For this review, take the finished solid that the model builds, in its own axes (mm). A direction names the side the tool comes from. Round coordinates to 2 decimals unless told otherwise and drop trailing zeros. Order: outer loops, then holes, each group sorted by start corner. A loop starts at its lowest first (then second) coordinate and runs counter-clockwise, first axis right, second up. Notation, with made-up numbers: M 82.5,34 L 121.5,34 A23 cw 121.5,62 Z; hole C 14,21 d4. An arc over 180 degrees is marked long. Put each result on its own line as item: value.
Autodesk Inventor part; units mm, degrees
ref_plane "YZ Plane" through (0, 0, 0) normal (1, 0, 0) x (0, 1, 0)
ref_plane "XZ Plane" through (0, 0, 0) normal (0, 1, 0) x (-1, 0, 0)
ref_plane "XY Plane" through (0, 0, 0) normal (0, 0, 1) x (1, 0, 0)
sketch "Sketch1" plane through (0, 0, 0) normal (1, 0, 0) x (0, 1, 0)
  line L0 (27.1, -22.6) -> (-27.1, -22.6)
  line L1 (-27.1, -22.6) -> (-27.1, 22.6)
  line L2 (-27.1, 22.6) -> (27.1, 22.6)
  line L3 (27.1, 22.6) -> (27.1, -22.6)
  line L4 (27.1, -22.6) -> (-27.1, 22.6) construction
  line L5 (-27.1, -22.6) -> (27.1, 22.6) construction
  point P0 (0, 0)
  dimension "d0" = 54.2
  dimension "d1" = 45.2
extrude "Extrusion1" add sketch "Sketch1" along normal blind 15.3
sketch "Sketch2" plane through (0, 27.1, 22.6) normal (0, 1, 0) x (1, 0, 0)
  line L0 (15.3, 0) -> (15.3, 45.2)
  line L1 (0, 0) -> (0, 45.2)
  line L2 (15.3, 0) -> (0, 0)
  line L3 (0, 0) -> (0, 45.2)
  line L4 (0, 45.2) -> (15.3, 45.2)
  line L5 (15.3, 45.2) -> (15.3, 0)
  point P0 (0, 22.6)
extrude "Extrusion2" add sketch "Sketch2" along normal blind 7
sketch "Sketch3" plane through (0, -27.1, -22.6) normal (0, -1, 0) x (1, 0, 0)
  line L0 (0, 45.2) -> (0, 0)
  line L1 (15.3, 45.2) -> (15.3, 0)
  line L2 (0, 45.2) -> (15.3, 45.2)
  line L3 (15.3, 45.2) -> (15.3, 0)
  line L4 (15.3, 0) -> (0, 0)
  line L5 (0, 0) -> (0, 45.2)
  point P0 (0, 22.6)
extrude "Extrusion3" add sketch "Sketch3" along normal blind 7
sketch "Sketch4" plane through (15.3, 0, 0) normal (1, 0, 0) x (0, 0, -1)
  line L0 (-22.6, -34.1) -> (-22.6, 34.1)
  line L1 (-22.6, 34.1) -> (22.6, 34.1)
  line L2 (-22.6, -34.1) -> (22.6, -34.1)
  line L3 (22.6, -34.1) -> (22.6, 34.1)
  line L4 (22.6, 34.1) -> (-22.6, 34.1)
  line L5 (-22.6, 34.1) -> (-22.6, -34.1)
  point P0 (0, 0)
extrude "Extrusion4" add sketch "Sketch4" along normal blind 7
sketch "Sketch5" plane through (0, 0, 0) normal (-1, 0, 0) x (0, 0, 1)
  line L0 (-22.6, 34.1) -> (22.6, 34.1)
  line L1 (22.6, -34.1) -> (-22.6, -34.1)
  line L2 (22.6, 34.1) -> (-22.6, 34.1)
  line L3 (-22.6, 34.1) -> (-22.6, -34.1)
  line L4 (-22.6, -34.1) -> (22.6, -34.1)
  line L5 (22.6, -34.1) -> (22.6, 34.1)
  point P0 (0, 0)
extrude "Extrusion5" add sketch "Sketch5" along normal blind 7
sketch "Sketch6" plane through (22.3, -34.1, -22.6) normal (0, 0, -1) x (-1, 0, 0)
  line L0 (29.3, 0) -> (0, 0)
  line L1 (0, 68.2) -> (0, 0)
  line L2 (29.3, 0) -> (0, 0)
  line L3 (0, 0) -> (0, 68.2)
  line L4 (0, 68.2) -> (29.3, 68.2)
  line L5 (29.3, 68.2) -> (29.3, 0)
  point P0 (22.3, 34.1)
extrude "Extrusion6" add sketch "Sketch6" along normal blind 10
sketch "Sketch7" plane through (-7, 0, 0) normal (-1, 0, 0) x (0, 0, 1)
  line L0 (22.6, 34.1) -> (-32.6, 34.1)
  line L1 (22.6, -34.1) -> (-32.6, -34.1)
  line L2 (-32.6, 34.1) -> (-22.6, 34.1)
  line L3 (-22.6, 34.1) -> (-22.6, -34.1)
  line L4 (-22.6, -34.1) -> (-32.6, -34.1)
  line L5 (-32.6, -34.1) -> (-32.6, 34.1)
  point P0 (0, 0)
  dimension "d14" = 10
extrude "Extrusion7" add sketch "Sketch7" along normal blind 20
sketch "Sketch8" plane through (22.3, -34.1, 22.6) normal (0, 0, 1) x (1, 0, 0)
  line L0 (0, 68.2) -> (-49.3, 68.2)
  line L1 (-29.3, 0) -> (-29.3, 68.2)
  line L2 (0, 68.2) -> (-29.3, 68.2)
  line L3 (-29.3, 68.2) -> (-29.3, 0)
  line L4 (-29.3, 0) -> (0, 0)
  line L5 (0, 0) -> (0, 68.2)
  line L6 (-22.25, 7) -> (-7.05, 7)
  line L7 (-7.05, 7) -> (-7.05, 61.2)
  line L8 (-7.05, 61.2) -> (-22.25, 61.2)
  line L9 (-22.25, 61.2) -> (-22.25, 7)
  line L10 (-22.25, 7) -> (-7.05, 61.2) construction
  line L11 (-7.05, 7) -> (-22.25, 61.2) construction
  point P0 (-22.3, 34.1)
  point P1 (-14.65, 34.1)
  dimension "d17" = 15.2
  dimension "d18" = 54.2
extrude "Extrusion8" cut sketch "Sketch8" against normal blind 45.2 contours L9 L8 L7 L6
sketch "Sketch9" plane through (22.3, 0, 0) normal (1, 0, 0) x (0, 0, -1)
  line L0 (-22.6, -27.1) -> (22.6, -27.1)
  line L1 (-22.6, 27.1) -> (22.6, 27.1)
  line L2 (-22.6, -27.1) -> (22.6, -27.1)
  line L3 (22.6, -27.1) -> (22.6, 27.1)
  line L4 (22.6, 27.1) -> (-22.6, 27.1)
  line L5 (-22.6, 27.1) -> (-22.6, -27.1)
  line L6 (-22.6, -27.1) -> (-5.1, -27.1)
  circle A0 centre (-5.1, -13.7) radius 2.1
  circle A1 centre (-5.1, -0.2) radius 2.1
  circle A2 centre (-5.1, 13.4) radius 2.1
  circle A3 centre (12.4, -13.7) radius 2.1
  circle A4 centre (12.4, -0.2) radius 2.1
  circle A5 centre (12.4, 13.4) radius 2.1
  point P0 (0, 0)
extrude "Extrusion9" cut sketch "Sketch9" against normal blind 39.25 contours A0 | A1 | A2 | A3 | A4 | A5
sketch "Sketch10" plane through (22.3, 0, 0) normal (1, 0, 0) x (0, 0, -1)
  line L0 (-22.6, -34.1) -> (32.6, -34.1)
  line L1 (-22.6, 34.1) -> (32.6, 34.1)
  line L2 (32.6, -34.1) -> (22.6, -34.1)
  line L3 (22.6, -34.1) -> (22.6, 34.1)
  line L4 (22.6, 34.1) -> (32.6, 34.1)
  line L5 (32.6, 34.1) -> (32.6, -34.1)
  point P0 (0, 0)
  dimension "d36" = 10
extrude "Extrusion10" add sketch "Sketch10" along normal blind 20
sketch "Sketch11" plane through (42.3, 0, 0) normal (1, 0, 0) x (0, 0, -1)
  line L0 (32.6, 73) -> (22.6, 73)
  line L1 (22.6, 73) -> (22.6, -73)
  line L2 (22.6, -73) -> (32.6, -73)
  line L3 (32.6, -73) -> (32.6, 73)
  line L4 (32.6, 73) -> (22.6, -73) construction
  line L5 (22.6, 73) -> (32.6, -73) construction
  point P0 (0, 0)
  point P1 (27.6, 0)
  dimension "d62" = 10
  dimension "d63" = 146
sketch "Sketch12" plane through (22.3, 0, 0) normal (1, 0, 0) x (0, 0, -1)
  circle A0 centre (-5.1, -0.2) radius 2.1
  circle A1 centre (12.4, -0.2) radius 2.1
  line L0 (-5.1, -0.2) -> (12.4, -0.2)
  line L1 (-22.6, 27.1) -> (22.6, 27.1)
  line L2 (-0.85, -27.5) -> (8.15, -27.5)
  line L3 (8.15, -27.5) -> (8.15, 27.1)
  line L4 (8.15, 27.1) -> (-0.85, 27.1)
  line L5 (-0.85, 27.1) -> (-0.85, -27.5)
  line L6 (-0.85, -27.5) -> (8.15, 27.1) construction
  line L7 (8.15, -27.5) -> (-0.85, 27.1) construction
  point P0 (0, 0)
  point P1 (3.65, -0.2)
  dimension "d42" = 9
extrude "Extrusion12" add sketch "Sketch12" along normal blind 15 contours L5 L1 L3 L0 | L0 L3 L2 L5
sketch "Sketch13" plane through (22.3, -27.5, 0.85) normal (0, 0, 1) x (1, 0, 0)
  line L0 (0, 0) -> (15, 0)
  line L1 (15, 0) -> (15, 10)
  line L2 (15, 54.6) -> (15, 0)
  line L3 (15, 0) -> (25, 0) construction
  line L4 (0, 54.6) -> (15, 54.6)
  line L5 (15, 54.6) -> (15, 44.6)
  line L6 (0, 54.6) -> (0, 0)
  line L7 (5, 10) -> (5, 44.6)
  line L8 (0, 44.6) -> (0, 10)
  line L9 (0, -6.6) -> (0, 3.4)
  line L10 (0, 61.6) -> (0, 51.6)
  line L11 (0, 61.6) -> (10, 61.6) construction
  line L12 (0, 3.4) -> (5, 3.4)
  line L13 (5, 3.4) -> (5, 51.6)
  line L14 (5, 51.6) -> (0, 51.6)
  line L15 (0, 51.6) -> (0, 3.4)
  point P0 (-22.3, 27.5)
  dimension "d45" = 10
  dimension "d46" = 90
  dimension "d47" = 10
  dimension "d48" = 5
  dimension "d56" = 10
  dimension "d57" = 10
  dimension "d58" = 90
sketch "Sketch14" plane through (22.3, 27.1, 0.85) normal (0, 1, 0) x (1, 0, 0)
  line L0 (15, 9) -> (15, 0)
  line L1 (0, 9) -> (0, 0)
  line L2 (15, 0) -> (0, 0)
  line L3 (0, 0) -> (0, 9)
  line L4 (0, 9) -> (15, 9)
  line L5 (15, 9) -> (15, 0)
  point P0 (-22.3, 0.85)
extrude "Extrusion14" add sketch "Sketch14" along normal blind 7
sketch "Sketch15" plane through (22.3, -27.5, -8.15) normal (0, -1, 0) x (1, 0, 0)
  line L0 (0, 0) -> (0, 9)
  line L1 (15, 9) -> (15, 0)
  line L2 (0, 9) -> (15, 9)
  line L3 (15, 9) -> (15, 0)
  line L4 (15, 0) -> (0, 0)
  line L5 (0, 0) -> (0, 9)
  point P0 (-22.3, 8.15)
extrude "Extrusion15" add sketch "Sketch15" along normal blind 7
extrude "Extrusion16" cut sketch "Sketch13" against normal blind 9.75 contours L6 L14 L13 L7 L12
fillet "Fillet2" radius 4.5 2 edges at (27.3, 0, 0.85) (27.3, 0, -8.15)
extrude "Extrusion17" add sketch "Sketch11" along normal blind 20
sketch "Sketch16" plane through (22.3, -34.1, -22.6) normal (0, 0, 1) x (1, 0, 0)
  line L0 (20, 0) -> (20, -38.9)
  line L1 (40, -38.9) -> (40, 107.1)
  line L2 (20, -38.9) -> (40, -38.9)
  line L3 (40, -38.9) -> (40, 107.1)
  line L4 (40, 107.1) -> (20, 107.1)
  line L5 (20, 107.1) -> (20, -38.9)
  line L6 (20, -38.9) -> (20, -18.9)
  line L7 (20, -18.9) -> (40, -18.9)
  line L8 (40, -18.9) -> (40, -38.9)
  line L9 (20, 107.1) -> (20, 87.1)
  line L10 (20, 68.2) -> (20, 107.1)
  line L11 (20, 87.1) -> (40, 87.1)
  line L12 (40, 107.1) -> (40, 87.1)
  line L13 (40, 107.1) -> (20, 107.1)
  line L14 (40, -18.9) -> (30, -18.9)
  line L15 (30, -18.9) -> (30, 87.1)
  line L16 (30, 87.1) -> (40, 87.1)
  line L17 (40, 87.1) -> (40, -18.9)
  point P0 (-22.3, 34.1)
  dimension "d66" = 20
  dimension "d67" = 20
  dimension "d68" = 10
extrude "Extrusion18" add sketch "Sketch16" along normal blind 20 contours L15 L11 L1 L7
sketch "Sketch17" plane through (62.3, 0, 0) normal (1, 0, 0) x (0, 0, -1)
  line L0 (2.6, -53) -> (2.6, 53)
  line L1 (22.6, -53) -> (2.6, -53)
  line L2 (2.6, -53) -> (22.6, -53)
  line L3 (22.6, 53) -> (2.6, 53)
  line L4 (22.6, -53) -> (22.6, 53)
  line L5 (2.6, 53) -> (2.6, 43)
  line L6 (2.6, 43) -> (2.6, 22)
  line L7 (2.6, -53) -> (2.6, -43)
  line L8 (2.6, -43) -> (2.6, -22)
  line L9 (2.6, 22) -> (2.6, 8)
  line L10 (2.6, -43) -> (12.6, -43)
  circle A0 centre (12.6, -43) radius 1.5
  circle A1 centre (12.6, -22) radius 1.5
  circle A2 centre (12.6, 8) radius 1.5
  circle A3 centre (12.6, 22) radius 1.5
  circle A4 centre (12.6, 43) radius 1.5
  line L11 (2.6, -53) -> (7.6, -53)
  line L12 (7.6, -53) -> (7.6, 53)
  line L13 (7.6, 53) -> (2.6, 53)
  line L14 (2.6, 53) -> (2.6, -53)
  point P0 (0, 0)
  dimension "d71" = 10
  dimension "d72" = 21
  dimension "d73" = 10
  dimension "d74" = 21
  dimension "d75" = 14
  dimension "d76" = 3
  dimension "d77" = 3
  dimension "d78" = 3
  dimension "d79" = 3
  dimension "d80" = 3
  dimension "d81" = 5
extrude "Extrusion19" cut sketch "Sketch17" against normal blind 20 contours L0 L10 L12 L1 | L0 L3 L12 L10 | A0 | A1 | A2 | A3 | A4
sketch "Sketch18" plane through (62.3, -53, -7.6) normal (0, 0, 1) x (1, 0, 0)
  line L0 (0, 0) -> (-10, 0)
  line L1 (0, 106) -> (0, 0)
  line L2 (-10, 0) -> (0, 0)
  line L3 (0, 0) -> (0, 106)
  line L4 (0, 106) -> (-10, 106)
  line L5 (-10, 106) -> (-10, 0)
  point P0 (-62.3, 53)
extrude "Extrusion20" add sketch "Sketch18" along normal blind 1.5
sketch "Sketch19" plane through (22.3, -34.1, -22.6) normal (0, 0, 1) x (1, 0, 0)
  line L0 (20, 107.1) -> (40, 107.1)
  line L1 (30, 107.1) -> (30, 97.1)
  line L2 (20, -38.9) -> (40, -38.9)
  line L3 (30, -38.9) -> (30, -28.9)
  line L4 (-29.3, 0) -> (-49.3, 0)
  line L5 (-39.3, 0) -> (-39.3, 68.2)
  line L6 (-29.3, 68.2) -> (-49.3, 68.2)
  line L7 (-39.3, 68.2) -> (-39.3, 53.2)
  line L8 (-39.3, 0) -> (-39.3, 15)
  line L9 (-39.3, 34.1) -> (-41.2293, 34.1)
  point P0 (-22.3, 34.1)
  dimension "d86" = 10
  dimension "d87" = 10
  dimension "d88" = 15
  dimension "d89" = 15
hole "Hole1" at (-17, 19.1, -22.6) at (-17, 0, -22.6) at (-17, -19.1, -22.6) at (52.3, 63, -22.6) at (52.3, -63, -22.6) direction (0, 0, -1) diameter 5 end through all countersink diameter 10 countersink angle 90
sketch "Sketch21" plane through (62.3, 0, 0) normal (1, 0, 0) x (0, 0, -1)
  line L0 (22.6, -73) -> (32.6, -73)
  line L1 (32.6, 73) -> (22.6, 73)
  line L2 (32.6, -73) -> (30.6, -73)
  line L3 (30.6, -73) -> (30.6, 73)
  line L4 (30.6, 73) -> (32.6, 73)
  line L5 (32.6, 73) -> (32.6, -73)
  point P0 (0, 0)
  dimension "d97" = 2
extrude "Extrusion21" cut sketch "Sketch21" against normal blind 171.5
properties part number "base"
(1) For faces 4 (the face through (28.653, 0.337, -6.867)), 5 (the face through (0.05, 0, 0)), 6 (the face through (33, 0, -8.15)), 7 (the face through (-3.43, 11.35, -11.94)), 8 (the face through (57, 53, -14)), list the 3-axis set-ups (+Z, -Z, +X, -X, +Y, -Y) from which the entire face can be reached by the end or side of a thin tool; tool diameter is ignored.
A:
face 4: none
face 5: +Z
face 6: +Y, -Y
face 7: -X
face 8: +Z, +X, -X, +Y
(2) Add section A-A on z = 5.1. State how many separate pieces and enclosed holes the cut face has, then the cut area to 3 significant figures.
A:
separate pieces: 6
enclosed holes: 0
area: 997 mm2
(3) Draft analysis for pull direction X (two halves, no side actions). For faces 1 (the face through (62.3, 1, -19)), 2 (the face through (52.4, -60.3, -24.9)), 3 (the face through (-3.43, 11.35, 5.56)), state which applies: released by +X, released by -X, zero draft, split by the parting line, or undercut.
A:
face 1: released by +X
face 2: undercut
face 3: zero draft
(4) Add section B-B on z = -19. Give the boundary of the cut face in (x, y), then the cut area to 3 significant figures.
A:
outline: M -7,-34.1 L 22.3,-34.1 L 22.3,34.1 L -7,34.1 Z; M 52.3,-53 L 62.3,-53 L 62.3,53 L 52.3,53 Z; hole M 0.05,-27.1 L 15.25,-27.1 L 15.25,27.1 L 0.05,27.1 Z
area: 2,230 mm2
(5) To check wall thickness, follow L1, parallel to Y at x = 17, z = 5.1; L2, parallel to Z at x = 20, y = 0; L3, parallel to Y at x = -17, z = -27.55. State the ranges of each line that lie inside material, in increasing order.
A:
L1: y = -34.1 to -15.8, -11.6 to -2.3, 1.9 to 11.3, 15.5 to 34.1
L2: z = -30.6 to -14.49, -10.31 to 3.01, 7.19 to 22.6
L3: y = -34.1 to -21.6, -16.6 to -2.5, 2.5 to 16.6, 21.6 to 34.1
(6) Add section D-D on x = 18.5. Give the boundary of the cut face in (y, z).
A:
outline: M -34.1,-30.6 L 34.1,-30.6 L 34.1,22.6 L -34.1,22.6 Z; hole C -13.7,-12.4 d4.2; hole C -13.7,5.1 d4.2; hole C -0.2,-12.4 d4.2; hole C -0.2,5.1 d4.2; hole C 13.4,-12.4 d4.2; hole C 13.4,5.1 d4.2
(7) Insertion check: pin 1 Ø4 at (y, z) = (-0.2, -12.4) entering from -X; pin 2 Ø6.5 at (y, z) = (44, -28.5) entering from -X; pin 3 Ø10 at (x, y) = (-14, 14) entering from +Z. Each pin has a flat end and moves straight along its axis. Give the tip position at first contact, or say it passes through.
A:
pin 1: stops at x = 52.3
pin 2: stops at x = 42.3
pin 3: stops at z = -22.6
(8) Add section C-C on y = 43. Give the boundary of the cut face in (x, z), then the cut area to 3 significant figures.
A:
outline: M 42.3,-30.6 L 62.3,-30.6 L 62.3,-14.1 L 52.3,-14.1 L 52.3,-22.6 L 42.3,-22.6 Z; M 52.3,-11.1 L 62.3,-11.1 L 62.3,-6.1 L 52.3,-6.1 Z
area: 295 mm2
